Can you work these out from the model? Positions are in its coordinate system, mm. Give positions to 0.01 mm unless a question says otherwise; leave off trailing zeros. Loops run counter-clockwise (first coordinate to the right, second up) from the corner with the lowest first, then second, coordinate; pieces in that order, holes last. Notation, with made-up numbers: (-29, -5) - (10, -5) arc R23 cw to (10, 12) - close; hole circle Ø11 at (-39.75, 22.5). An arc over 180 degrees is marked (long way). Write item = value, one per line.
from build123d import *

# Parameters (mm, degrees)
F0_W     = 304.8
F0_H     = 25.4
F2_DEPTH = 2
F1_R     = 6.35
F3_DEPTH = 108
F4_R     = 6.35
F5_DEPTH = 25.4


with BuildPart() as f2:
    # F0 (on Front) → F2 (new body)
    with BuildSketch(Plane.XZ):
        with Locations((-193.59771, 10.958225)):
            Rectangle(F0_W, F0_H)
    extrude(amount=-F2_DEPTH)

    # F1 (on face) → F3 (cut)
    with BuildSketch(Plane.XZ):
        with Locations((-209.174946, 10.958225)):
            Circle(F1_R)
    extrude(amount=-F3_DEPTH, mode=Mode.SUBTRACT)

    # F4 (on face) → F5 (cut)
    with BuildSketch(Plane.XZ):
        with Locations((-320.59771, 10.958225)):
            Circle(F4_R)
        with Locations((-66.59771, 10.958225)):
            Circle(F4_R)
    extrude(amount=-F5_DEPTH, mode=Mode.SUBTRACT)


solid = f2.part
Q1. Imagine slicing it at B-B, the plane x = -206. Write out the boundary of the cut face in (y, z), then the cut area to 3 significant figures.
Output:
outline = (0, -1.74) - (2, -1.74) - (2, 5.46) - (0, 5.46) - close; (0, 16.46) - (2, 16.46) - (2, 23.66) - (0, 23.66) - close
area = 28.8 mm2
Q2. I need wall thicknesses on L1, parallel to X at y = 0.95, z = 11.75; L2, parallel to X at y = 0.25, z = 11.25. Which ranges of each line are inside material? Lowest first, please.
Output:
L1 = -346 to -326.9, -314.3 to -215.48, -202.87 to -72.9, -60.3 to -41.2
L2 = -346 to -326.94, -314.25 to -215.52, -202.83 to -72.94, -60.25 to -41.2
Q3. We'd pull the mould along X, two halves only. Please class faces 1 (the cylindrical face through (-214.21, 0.99, 7.09)), 2 (the flat face through (-196, 2, 11)), 3 (the cylindrical face through (-325.637, 0.986, 7.094)): released by +X, released by -X, zero draft, split by the parting line, or undercut.
Output:
face_1 = undercut
face_2 = zero draft
face_3 = undercut
Q4. For pin 1 (11.5 mm diameter, centred on x = -320.6, z = 10.96, fed in from -Y), with a flat end and sliding along its axis, tell me the tip position at first contact or that it passes through.
Output:
pin_1 = through
Q5. Imagine slicing it at A-A, the plane y = 0.7. Write out the boundary of the cut face in (x, z), then the cut area to 3 significant figures.
Output:
outline = (-346, -1.74) - (-41.2, -1.74) - (-41.2, 23.66) - (-346, 23.66) - close; hole circle Ø12.7 at (-320.6, 10.96); hole circle Ø12.7 at (-209.17, 10.96); hole circle Ø12.7 at (-66.6, 10.96)
area = 7,360 mm2
